Build history of the part. All positions in model axes, mm. A direction names the side the tool comes from. Give positions to 0.01 mm unless a question says otherwise; leave off trailing zeros. Loops run counter-clockwise (first coordinate to the right, second up) from the corner with the lowest first, then second, coordinate; pieces in that order, holes last. Notation, with made-up numbers: M 20,7 L 32,7 A24 ccw 32,38 Z; hole C -16,79 d10. An arc over 180 degrees is marked long. Answer in a Markdown table with one row per item. Add a question column.
```python
from build123d import *

# Parameters (mm, degrees)
F1_DEPTH  = 533.4
F0_R      = 6.35
F2_DEPTH  = 50.8
F4_DEPTH  = 171.45
F6_DEPTH  = 165.1
F7_R      = 3.175
F8_DEPTH  = 88.9
F9_R      = 3.175
F10_DEPTH = 25.4
F11_R     = 3.175
F12_DEPTH = 25.4
F13_W     = 6.35
F13_H     = 6.35
F14_DEPTH = 533.4


# Not quite as in the source:
# - a feature names something its author has since deleted; it is built from what else it names


with BuildPart() as f1:
    # F0 (on Top) → F1 (new body)
    with BuildSketch(Plane.XY):
        Polygon((-171.45, 165.1), (-171.45, 0), (171.45, 0), (171.45, 165.1), (63.5, 165.1), (63.5, 114.3), (120.65, 114.3), (120.65, 50.8), (-120.65, 50.8), (-120.65, 114.3), (-63.5, 114.3), (-63.5, 165.1), align=None)
    extrude(amount=F1_DEPTH)

    # F0 (on Top) → F2 (join)
    with BuildSketch(Plane.XY):
        Polygon((-171.45, 165.1), (-171.45, 0), (171.45, 0), (171.45, 165.1), (63.5, 165.1), (63.5, 114.3), (120.65, 114.3), (120.65, 50.8), (-120.65, 50.8), (-120.65, 114.3), (-63.5, 114.3), (-63.5, 165.1), align=None)
        Polygon((171.45, 0), (-171.45, 0), (-171.45, 165.1), (-558.8, 165.1), (-558.8, -444.5), (558.8, -444.5), (558.8, 165.1), (171.45, 165.1), align=None)
        with Locations((-508, -393.7)):
            Circle(F0_R, mode=Mode.SUBTRACT)
        with Locations((508, -393.7)):
            Circle(F0_R, mode=Mode.SUBTRACT)
    extrude(amount=F2_DEPTH)

    # F3 (on Right) → F4 (join, symmetric)
    with BuildSketch(Plane.YZ):
        Polygon((-444.5, 50.8), (0, 50.8), (0, 533.4), align=None)
    extrude(amount=F4_DEPTH, both=True)

    # F5 (on face) → F6 (join)
    with BuildSketch(Plane(origin=(0, 165.1, 0), x_dir=(-1, 0, 0), z_dir=(0, 1, 0))):
        Polygon((-558.8, 50.8), (-171.45, 50.8), (-171.45, 533.4), align=None)
        Polygon((171.45, 533.4), (171.45, 50.8), (558.8, 50.8), align=None)
    extrude(amount=-F6_DEPTH)

    # F7 (on face) → F8 (cut, symmetric)
    with BuildSketch(Plane(origin=(0, 50.8, 0), x_dir=(-1, 0, 0), z_dir=(0, 1, 0))):
        with Locations((-89.2969816923, 146.05)):
            Circle(F7_R)
        with Locations((-89.2969816923, 266.7)):
            Circle(F7_R)
        with Locations((-89.2969816923, 25.4)):
            Circle(F7_R)
        with Locations((-89.2969816923, 508)):
            Circle(F7_R)
        with Locations((-89.2969816923, 387.35)):
            Circle(F7_R)
        with Locations((89.2969816923, 25.4)):
            Circle(F7_R)
        with Locations((89.2969816923, 146.05)):
            Circle(F7_R)
        with Locations((89.2969816923, 266.7)):
            Circle(F7_R)
        with Locations((89.2969816923, 387.35)):
            Circle(F7_R)
        with Locations((89.2969816923, 508)):
            Circle(F7_R)
    extrude(amount=F8_DEPTH, both=True, mode=Mode.SUBTRACT)

    # F9 (on face) → F10 (cut)
    with BuildSketch(Plane(origin=(120.65, 0, 0), x_dir=(0, -1, 0), z_dir=(-1, 0, 0))):
        with Locations((-82.55, 25.4)):
            Circle(F9_R)
        with Locations((-82.55, 146.05)):
            Circle(F9_R)
        with Locations((-82.55, 266.7)):
            Circle(F9_R)
        with Locations((-82.55, 387.35)):
            Circle(F9_R)
        with Locations((-82.55, 508)):
            Circle(F9_R)
    extrude(amount=-F10_DEPTH, mode=Mode.SUBTRACT)

    # F11 (on face) → F12 (cut)
    with BuildSketch(Plane.YZ.offset(-120.65)):
        with Locations((82.55, 25.4)):
            Circle(F11_R)
        with Locations((82.55, 146.05)):
            Circle(F11_R)
        with Locations((82.55, 266.7)):
            Circle(F11_R)
        with Locations((82.55, 387.35)):
            Circle(F11_R)
        with Locations((82.55, 508)):
            Circle(F11_R)
    extrude(amount=-F12_DEPTH, mode=Mode.SUBTRACT)

    # F13 (on Top) → F14 (join)
    with BuildSketch(Plane.XY):
        with Locations((-117.475, 53.975)):
            Rectangle(F13_W, F13_H)
    extrude(amount=F14_DEPTH)


solid = f1.part
```
(1) Pull direction X, two halves, no side cores. Call faces 1 (the flat face through (362, -219, 50.8)), 2 (the flat face through (5, 50.8, 263)), 3 (the flat face through (-558.8, -135, 25)), 4 (the flat face through (362.41, 83.71, 295.48)): +X half, -X half, draft (parallel to the pull), parting line (faces both ways), or undercut.
(2) Slice it at B-B, the plane z = 350. Give the cut face in (x, y).
(3) Slice it at C-C, the plane x = -8. Give the cut face in (y, z).
(4) Tool access for faces 5 (the flat face through (260, 165.1, 211)), 6 (the flat face through (92, 114.3, 263)), 7 (the flat face through (282, 0, 188)), 8 (the flat face through (-276, 0, 188)), 9 (the flat face through (63.5, 140, 263)): list every direction of +Z, -Z, +X, -X, +Y, -Y with a clear straight run to the whole face (end or side of a thin tool).
(5) Wall check: line 1 (X direction, y = -1.5, z = 146.05); line 2 (Z direction, x = -131.75, y = 82.55) (3 decimals); line 3 (X direction, y = 127.75, z = 25.4). Give the ranges that are in metal, low to high.
(6) Pin check, flat tips, straight feed: pin 1 (1 mm diameter, centred on x = 159.5, z = 370, fed in from -Y); pin 2 (10 mm diameter, centred on y = 82.55, z = 387.35, fed in from -X); pin 3 (3 mm diameter, centred on x = 88.5, z = 266, fed in from -Y). Stop position of each tip, or through.
(7) Slice it at A-A, the plane y = -296. Give the cut face in (x, z), then the cut area to 3 significant figures.
(8) Slice it at D-D, the plane y = -79. Give the cut face in (x, z), then the cut area to 3 significant figures.
Solution:
| question | item | result |
|---|---|---|
| 1 | face 1 | draft |
| 1 | face 2 | undercut |
| 1 | face 3 | -X half |
| 1 | face 4 | +X half |
| 2 | outline | M -318.65,0 L -171.45,0 L -171.45,-168.92 L 171.45,-168.92 L 171.45,0 L 318.65,0 L 318.65,165.1 L 63.5,165.1 L 63.5,114.3 L 120.65,114.3 L 120.65,50.8 L -114.3,50.8 L -114.3,57.15 L -120.65,57.15 L -120.65,114.3 L -63.5,114.3 L -63.5,165.1 L -318.65,165.1 Z |
| 3 | outline | M -444.5,0 L 50.8,0 L 50.8,533.4 L 0,533.4 L -444.5,50.8 Z |
| 4 | face 5 | +Z, -Z, +X, -X, +Y |
| 4 | face 6 | +Z, -Z |
| 4 | face 7 | +Z, +X, -Y |
| 4 | face 8 | +Z, -X, -Y |
| 4 | face 9 | +Z, -Z, +Y |
| 5 | line 1 | -171.45 to -92.47, -86.12 to 86.12, 92.47 to 171.45 |
| 5 | line 2 | 0 to 22.225, 28.575 to 142.875, 149.225 to 263.525, 269.875 to 384.175, 390.525 to 504.825, 511.175 to 533.4 |
| 5 | line 3 | -558.8 to -92.47, -86.12 to -63.5, 63.5 to 86.12, 92.47 to 558.8 |
| 6 | pin 1 | y = -150.96 |
| 6 | pin 2 | x = -292.69 |
| 6 | pin 3 | y = -247.67 |
| 7 | outline | M -558.8,0 L 558.8,0 L 558.8,50.8 L 171.45,50.8 L 171.45,212.03 L -171.45,212.03 L -171.45,50.8 L -558.8,50.8 Z |
| 7 | area | 112,000 mm^2 |
| 8 | outline | M -558.8,0 L 558.8,0 L 558.8,50.8 L 171.45,50.8 L 171.45,447.63 L -171.45,447.63 L -171.45,50.8 L -558.8,50.8 Z |
| 8 | area | 193,000 mm^2 |
